from build123d import *

# Parameters (mm, degrees)
SKETCH_1_W                  = 100
SKETCH_1_H                  = 160
EXTRUDE_1_DEPTH             = 4
SKETCH_2_R                  = 2
CUT_EXTRUDE_1_DEPTH         = 4
SKETCH_3_R                  = 1.5
CUT_EXTRUDE_2_DEPTH         = 4
SKETCH_4_R                  = 1.5
CUT_EXTRUDE_3_DEPTH         = 4
SKETCH_6_W                  = 100
SKETCH_6_H                  = 4
EXTRUDE_2_DEPTH             = 18
SKETCH_5_R                  = 1.5
CUT_EXTRUDE_4_DEPTH         = 10
PATTERN_LINEAR_1_COUNT      = 2
PATTERN_LINEAR_1_PITCH      = 20
PATTERN_LINEAR_1_COUNT_DIR2 = 2
PATTERN_LINEAR_1_PITCH_DIR2 = 15
MIRROR_3_COPY_1_SKETCH_R    = 1.5
MIRROR_3_COPY_1_DEPTH       = 10
MIRROR_3_COPY_2_SKETCH_R    = 1.5
MIRROR_3_COPY_2_DEPTH       = 10
MIRROR_3_COPY_3_SKETCH_R    = 1.5
MIRROR_3_COPY_3_DEPTH       = 10
FILLET_1_R                  = 10
SKETCH_7_R                  = 2
CUT_EXTRUDE_5_DEPTH         = 10


with BuildPart() as part:
    # 草图1 → 凸台-拉伸1 (new body)
    with BuildSketch(Plane(origin=(0, 0, 0), x_dir=(1, 0, 0), z_dir=(0, 1, 0))):
        Rectangle(SKETCH_1_W, SKETCH_1_H)
    extrude(amount=EXTRUDE_1_DEPTH)

    # 草图2 → 切除-拉伸1 (cut)
    with BuildSketch(Plane(origin=(0, 4, 0), x_dir=(1, 0, 0), z_dir=(0, 1, 0))):
        with Locations(Location((40, -3, 0), (0, 0, 270))):
            Circle(SKETCH_2_R)
        with Locations(Location((26, -3, 0), (0, 0, 270))):
            Circle(SKETCH_2_R)
        with Locations(Location((40, -35, 0), (0, 0, 90))):
            Circle(SKETCH_2_R)
        with Locations(Location((26, -35, 0), (0, 0, 90))):
            Circle(SKETCH_2_R)
    extrude(amount=-CUT_EXTRUDE_1_DEPTH, mode=Mode.SUBTRACT)

    # 草图3 → 切除-拉伸2 (cut)
    with BuildSketch(Plane(origin=(0, 4, 0), x_dir=(1, 0, 0), z_dir=(0, 1, 0))):
        with Locations(Location((-39, 44, 0), (0, 0, 270))):
            Circle(SKETCH_3_R)
        with Locations(Location((-11, 44, 0), (0, 0, 270))):
            Circle(SKETCH_3_R)
        with Locations(Location((-11, 16, 0), (0, 0, 270))):
            Circle(SKETCH_3_R)
        with Locations(Location((-39, 16, 0), (0, 0, 270))):
            Circle(SKETCH_3_R)
    cut_extrude_2 = extrude(amount=-CUT_EXTRUDE_2_DEPTH, mode=Mode.SUBTRACT)

    # 镜向1: 切除-拉伸2 across plane
    add(cut_extrude_2.mirror(Plane.XY), mode=Mode.SUBTRACT)

    # 草图4 → 切除-拉伸3 (cut)
    with BuildSketch(Plane(origin=(0, 4, 0), x_dir=(1, 0, 0), z_dir=(0, 1, 0))):
        with Locations(Location((42, 12, 0), (0, 0, 270))):
            Circle(SKETCH_4_R)
        with Locations(Location((8, 12, 0), (0, 0, 90))):
            Circle(SKETCH_4_R)
        with Locations(Location((42, -12, 0), (0, 0, 90))):
            Circle(SKETCH_4_R)
        with Locations(Location((8, -12, 0), (0, 0, 270))):
            Circle(SKETCH_4_R)
    extrude(amount=-CUT_EXTRUDE_3_DEPTH, mode=Mode.SUBTRACT)

    # 草图6 → 凸台-拉伸2 (add)
    with BuildSketch(Plane(origin=(0, 0, -80), x_dir=(-1, 0, 0), z_dir=(0, 0, -1))):
        with Locations((0, 2)):
            Rectangle(SKETCH_6_W, SKETCH_6_H)
    extrude_2 = extrude(amount=EXTRUDE_2_DEPTH)

    # 草图5 → 切除-拉伸4 (cut)
    with BuildSketch(Plane(origin=(0, 4, 0), x_dir=(1, 0, 0), z_dir=(0, 1, 0))):
        with Locations(Location((-35, 83, 0), (0, 0, 270))):
            Circle(SKETCH_5_R)
    cut_extrude_4 = extrude(amount=-CUT_EXTRUDE_4_DEPTH, mode=Mode.SUBTRACT)

    # 镜向2: 凸台-拉伸2 across plane
    add(extrude_2.mirror(Plane.XY))

    # 阵列(线性)1: Cut-Extrude 4 2 × 2
    with Locations(*[(j * PATTERN_LINEAR_1_PITCH_DIR2, 0, i * PATTERN_LINEAR_1_PITCH) for i in range(PATTERN_LINEAR_1_COUNT) for j in range(PATTERN_LINEAR_1_COUNT_DIR2) if (i, j) != (0, 0)]):
        add(cut_extrude_4, mode=Mode.SUBTRACT)

    # 镜向3: 切除-拉伸4 across plane
    add(cut_extrude_4.mirror(Plane.XY), mode=Mode.SUBTRACT)

    # 镜向3 copy 1 sketch → 镜向3 copy 1 (cut)
    with BuildSketch(Plane(origin=(15, 4, 0), x_dir=(1, 0, 0), z_dir=(0, 1, 0))):
        with Locations((-35, -83)):
            Circle(MIRROR_3_COPY_1_SKETCH_R)
    extrude(amount=-MIRROR_3_COPY_1_DEPTH, mode=Mode.SUBTRACT)

    # 镜向3 copy 2 sketch → 镜向3 copy 2 (cut)
    with BuildSketch(Plane(origin=(0, 4, -20), x_dir=(1, 0, 0), z_dir=(0, 1, 0))):
        with Locations((-35, -83)):
            Circle(MIRROR_3_COPY_2_SKETCH_R)
    extrude(amount=-MIRROR_3_COPY_2_DEPTH, mode=Mode.SUBTRACT)

    # 镜向3 copy 3 sketch → 镜向3 copy 3 (cut)
    with BuildSketch(Plane(origin=(15, 4, -20), x_dir=(1, 0, 0), z_dir=(0, 1, 0))):
        with Locations((-35, -83)):
            Circle(MIRROR_3_COPY_3_SKETCH_R)
    extrude(amount=-MIRROR_3_COPY_3_DEPTH, mode=Mode.SUBTRACT)

    # 圆角1
    fillet_1_edges = [part.edges().sort_by_distance(p)[0] for p in [
        (50, 2, 98),
        (-50, 2, 98),
        (50, 2, -98),
        (-50, 2, -98),
    ]]
    fillet(fillet_1_edges, radius=FILLET_1_R)

    # 草图7 → 切除-拉伸5 (cut)
    with BuildSketch(Plane(origin=(0, 4, 0), x_dir=(1, 0, 0), z_dir=(0, 1, 0))):
        with Locations(Location((-44, 37.5, 0), (0, 0, 270))):
            Circle(SKETCH_7_R)
        with Locations(Location((-4, 37.5, 0), (0, 0, 270))):
            Circle(SKETCH_7_R)
        with Locations(Location((-4, -37.5, 0), (0, 0, 270))):
            Circle(SKETCH_7_R)
        with Locations(Location((-44, -37.5, 0), (0, 0, 270))):
            Circle(SKETCH_7_R)
    extrude(amount=-CUT_EXTRUDE_5_DEPTH, mode=Mode.SUBTRACT)


solid = part.part
Could you check a few things on this model? Use its own coordinates, in mm. Coordinates: 2 decimals unless noted, no trailing zeros. Write each loop counter-clockwise with the first axis right and the second up, starting at its lowest first coordinate (ties: lowest second). Pieces come first, ordered by that corner, then holes. Notation, with made-up numbers: (54, 30) - (110, 30) arc R17 ccw to (110, 47) - close; hole circle Ø8 at (85.5, 77.25). An arc over 180 degrees is marked (long way). Put each result on its own line as item: value. Start each with the question number.
Q1. I want a section at A-A on z = -37.5. Write out the boundary of the cut face in (x, y), plus the area to 3 significant figures.
Q2. Please list where these lines run through material, in increasing order: L1, parallel to X at y = 1.15, z = -44; L2, parallel to X at y = 2.3, z = -63; L3, parallel to Z at x = -19.5, y = 0.6.
Q3. I want a section at B-B on y = 2.6. Count the separate pieces of the cut face and the enclosed holes in it, plus the area to 3 significant figures.
Q4. Thinking about a two-plate mould opening in X: for faces 1 (the cylindrical face through (-46.99, 2.03, 95.15)), 2 (the flat face through (50, 2, -1)), 3 (the cylindrical face through (-45.952, 2.028, -37.934)), which applies, pulls with the +X half, pulls with the -X half, needs draft (parallel to the pull), parting line crosses it, or undercut?
Checks:
1. outline: (-50, 0) - (-46, 0) - (-46, 4) - (-50, 4) - close; (-42, 0) - (-6, 0) - (-6, 4) - (-42, 4) - close; (-2, 0) - (50, 0) - (50, 4) - (-2, 4) - close
1. area: 368 mm²
2. L1: -50 to -40.5, -37.5 to -12.5, -9.5 to 50
2. L2: -50 to -36.5, -33.5 to -21.5, -18.5 to 50
2. L3: -98 to -84.41, -81.59 to -64.41, -61.59 to 61.59, 64.41 to 81.59, 84.41 to 98
3. separate pieces: 1
3. enclosed holes: 28
3. area: 19,300 mm²
4. face 1: pulls with the -X half
4. face 2: pulls with the +X half
4. face 3: undercut
